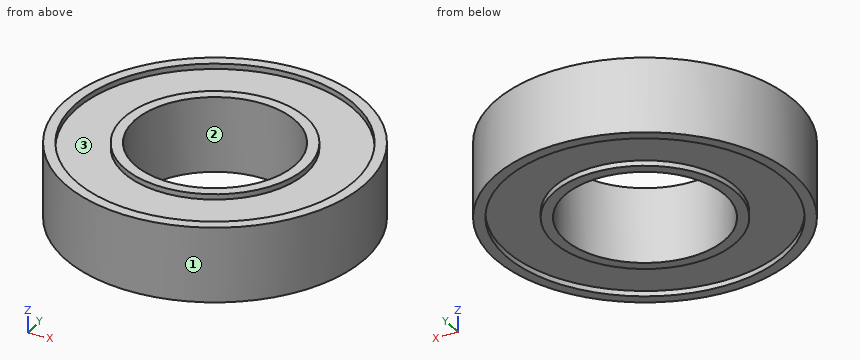
Autodesk Inventor part; units mm, degrees
ref_plane "Work Plane1" through (0, 0, 3.5) normal (0, 0, 1) x (1, 0, 0)
ref_plane "YZ Plane" through (0, 0, 0) normal (1, 0, 0) x (0, 1, 0)
ref_plane "XZ Plane" through (0, 0, 0) normal (0, 1, 0) x (-1, 0, 0)
sketch "Sketch1" plane through (0, 0, 0) normal (0, 0, 1) x (1, 0, 0)
  circle A0 centre (0, 0) radius 7.5
  circle A1 centre (0, 0) radius 14
  dimension "d0" = 15
  dimension "d1" = 28
extrude "Extrusion1" add sketch "Sketch1" along normal blind 7
sketch "Sketch2" plane through (0, 0, 7) normal (0, 0, 1) x (1, 0, 0)
  circle A0 centre (0, 0) radius 14
  circle A1 centre (0, 0) radius 7.5
  circle A2 centre (0, 0) radius 8.5
  circle A3 centre (0, 0) radius 13
  dimension "d4" = 1
  dimension "d5" = 1
extrude "Extrusion2" cut sketch "Sketch2" against normal blind 0.5 contours A3
ref_plane "Work Plane1" through (0, 0, 3.5) normal (0, 0, 1) x (1, 0, 0)
mirror "Mirror1" about plane through (0, 0, 3.5) normal (0, 0, 1) of "Extrusion2"
properties part number "6901 Bearing"
Part model, mm, in its own coordinate system. Face numbers are marked on the shaded views. Give positions to 0.01 mm unless a question says otherwise; leave off trailing zeros. Write each loop counter-clockwise with the first axis right and the second up, starting at its lowest first coordinate (ties: lowest second). Pieces come first, ordered by that corner, then holes. Notation, with made-up numbers: (17, 9.5) -> (39, 9.5) arc R19 cw to (39, 13.5) -> close; hole circle Ø8 at (23, 70). An arc over 180 degrees is marked (long way). Put each result on its own line as item: value. Start each with the question number.
Item 1: Cut at A-A (x = 0). List the corners of the cut face in (y, z).
Item 2: Wall check: L1, parallel to Y at x = 0, z = 0.3; L2, parallel to Y at x = 0, z = 3. Give the ranges that are in metal, low to high. Write a range as [from, to].
Item 3: Pin check, flat tips, straight feed: pin 1 Ø2 at (x, y) = (1.5, -5) entering from +Z; pin 2 Ø1.5 at (y, z) = (-9.5, 1) entering from -X; pin 3 Ø4 at (y, z) = (10, 3.5) entering from -X; pin 4 Ø1 at (x, z) = (7, 2) entering from -Y. Stop position of each tip, or through.
Item 4: Cut at C-C (z = 2.75). List the corners of the cut face in (x, y).
Item 5: Pull direction Y, two halves, no side cores. Call the marked faces 1, 2 and 3: pulls with the +Y half, pulls with the -Y half, needs draft (parallel to the pull), parting line crosses it, or undercut.
Item 6: Cut at D-D (y = 9.25). List the corners of the cut face in (x, z).
Answer list:
1. outline: (-14, 0) -> (-13, 0) -> (-13, 0.5) -> (-8.5, 0.5) -> (-8.5, 0) -> (-7.5, 0) -> (-7.5, 7) -> (-8.5, 7) -> (-8.5, 6.5) -> (-13, 6.5) -> (-13, 7) -> (-14, 7) -> close; (7.5, 0) -> (8.5, 0) -> (8.5, 0.5) -> (13, 0.5) -> (13, 0) -> (14, 0) -> (14, 7) -> (13, 7) -> (13, 6.5) -> (8.5, 6.5) -> (8.5, 7) -> (7.5, 7) -> close
2. L1: y = [-14, -13], [-8.5, -7.5], [7.5, 8.5], [13, 14]
2. L2: y = [-14, -7.5], [7.5, 14]
3. pin 1: passes through
3. pin 2: stops at x = -10.93
3. pin 3: stops at x = -11.49
3. pin 4: stops at y = -12.4
4. outline: circle Ø28 at (0, 0); hole circle Ø15 at (0, 0)
5. face 1: parting line crosses it
5. face 2: undercut
5. face 3: undercut
6. outline: (-10.51, 0) -> (-9.13, 0) -> (-9.13, 0.5) -> (9.13, 0.5) -> (9.13, 0) -> (10.51, 0) -> (10.51, 7) -> (9.13, 7) -> (9.13, 6.5) -> (-9.13, 6.5) -> (-9.13, 7) -> (-10.51, 7) -> close
